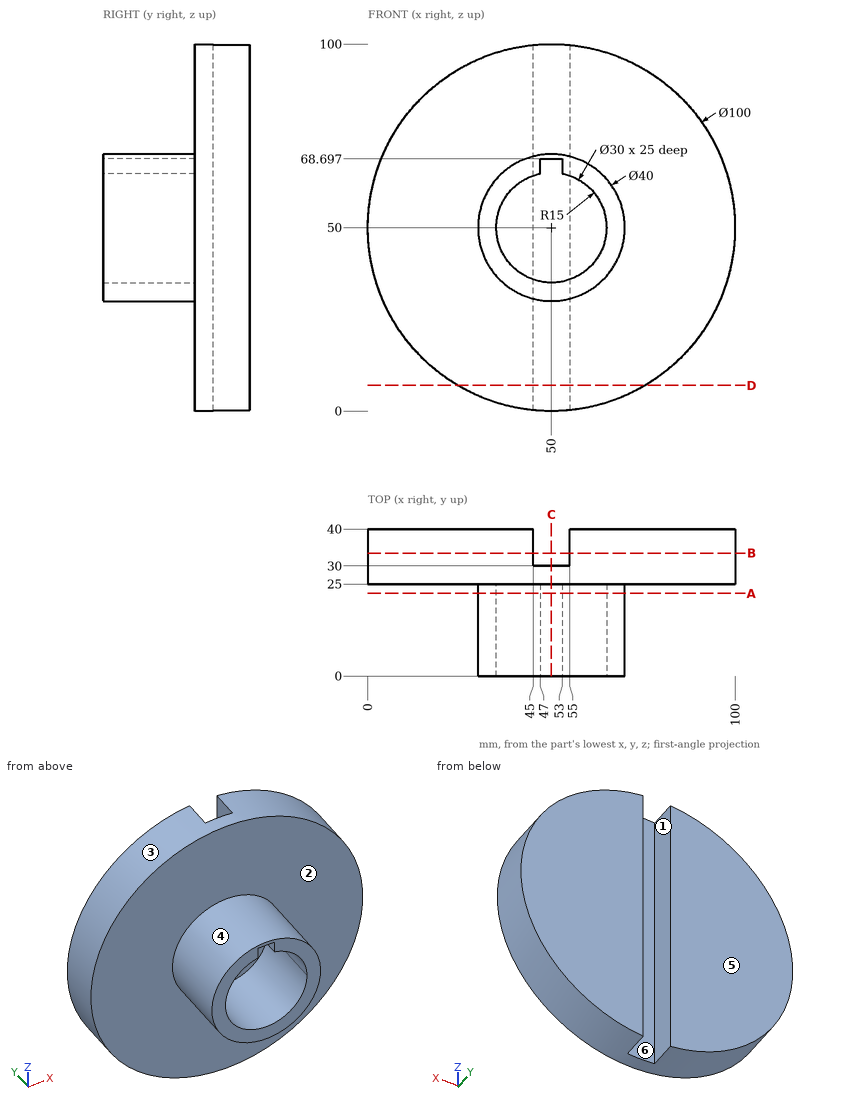
The drawing under review shows one solid part. Ordinate dimensions are in mm from its lowest x, y, z. A direction names the side the tool comes from. Coordinates: 2 decimals unless noted, no trailing zeros. Write each loop counter-clockwise with the first axis right and the second up, starting at its lowest first coordinate (ties: lowest second). Pieces come first, ordered by that corner, then holes. Notation, with made-up numbers: (61, 41.5) - (100, 41.5) arc R27 ccw to (100, 60.5) - close; hole circle Ø4 at (69.5, 16.5). An arc over 180 degrees is marked (long way). Answer in a Markdown table with one row per item. Add a question column.
Q1. We need section A-A, the plane y = 22.5. State the section outline as (x, z) points, and give its area (3 significant figures).
Q2. We need section C-C, the plane x = 50. State the section outline as (y, z) points, and give its area (3 significant figures).
Q3. We need section B-B, the plane y = 33.5. State the section outline as (x, z) points, and give its area (3 significant figures).
Q4. Draft analysis for pull direction X (two halves, no side actions). For the marked faces 4, 5 and 6, state which applies: +X half, -X half, draft (parallel to the pull), parting line (faces both ways), or undercut.
Q5. For probe 1 along X at (y, z) = (19, 50); probe 2 along Y at (x, z) = (47, 11); probe 3 along Y at (x, z) = (71.5, 57), list the stretches that pass through material, from the lowest coordinate up.
Q6. Tool access review of the marked faces 1, 2 and 3: name each direction out of +Z, -Z, +X, -X, +Y, -Y from which nothing blocks a thin tool from reaching the whole face with its end or side.
Q7. We need section D-D, the plane z = 7. State the section outline as (x, y) points.
Q8. For P1, Ø4, axis at y = 11.5, z = 38, coming from the -X side; P2, Ø3, axis at y = 18.5, z = 66, coming from the +X side (3 decimals); P3, Ø11, axis at y = 35.5, z = 70, coming from the +X side, all flat-tipped, find the tip position at first contact; note any pin that passes through.
Answer list:
| question | item | result |
|---|---|---|
| 1 | outline | circle Ø40 at (50, 50); hole (47, 64.7) arc R15 ccw (long way) to (53, 64.7) - (53, 68.7) - (47, 68.7) - close |
| 1 | area | 527 mm2 |
| 2 | outline | (0, 30) - (25, 30) - (25, 0) - (30, 0) - (30, 100) - (25, 100) - (25, 70) - (0, 70) - (0, 68.7) - (25, 68.7) - (25, 35) - (0, 35) - close |
| 2 | area | 658 mm2 |
| 3 | outline | (45, 0.25) - (45, 99.75) arc R50 ccw to start; (55, 0.25) arc R50 ccw to (55, 99.75) - close |
| 3 | area | 6,860 mm2 |
| 4 | face 4 | parting line |
| 4 | face 5 | draft |
| 4 | face 6 | undercut |
| 5 | probe 1 | x = 30 to 35, 65 to 70 |
| 5 | probe 2 | y = 25 to 30 |
| 5 | probe 3 | y = 25 to 40 |
| 6 | face 1 | +Z, -Z, +Y |
| 6 | face 2 | -Y |
| 6 | face 3 | +Y, -Y |
| 7 | outline | (24.49, 25) - (75.51, 25) - (75.51, 40) - (55, 40) - (55, 30) - (45, 30) - (45, 40) - (24.49, 40) - close |
| 8 | P1 | stops at x = 32.68 |
| 8 | P2 | stops at x = 63.775 |
| 8 | P3 | stops at x = 97.85 |
